Could you check a few things on this model? Use its own coordinates, in mm. Coordinates: 2 decimals unless noted, no trailing zeros. Order: outer loops, then holes, each group sorted by start corner. A loop starts at its lowest first (then second) coordinate and runs counter-clockwise, first axis right, second up. Notation, with made-up numbers: (19.25, 14.5) - (68.25, 14.5) arc R23 cw to (68.25, 26.5) - close; hole circle Ø4 at (-38, -23.5). An arc over 180 degrees is marked (long way). One line per item, written item: value.
from build123d import *

# Parameters (mm, degrees)
EXTRUDE_1_DEPTH     = 2
FILLET_1_R          = 5
FILLET_2_R          = 2
SKETCH_2_R          = 1.55
CUT_EXTRUDE_1_DEPTH = 2


with BuildPart() as part:
    # 草图1 → 凸台-拉伸1 (new body)
    with BuildSketch(Plane.XY):
        Polygon((387.201278127, -62.835808376), (387.201278127, 41.164191624), (257.201278127, 41.164191624), (213.03572495, 25.089244888), (173.136911199, -10.835808376), (213.03572495, -46.760861639), (257.201278127, -62.835808376), align=None)
    extrude(amount=EXTRUDE_1_DEPTH)

    # 圆角1
    fillet_1_edges = [part.edges().sort_by_distance(p)[0] for p in [
        (173.136911199, -10.835808376, 1),
    ]]
    fillet(fillet_1_edges, radius=FILLET_1_R)

    # 圆角2
    fillet_2_edges = [part.edges().sort_by_distance(p)[0] for p in [
        (257.201278127, -62.835808376, 1),
        (213.03572495, -46.760861639, 1),
        (213.03572495, 25.089244888, 1),
        (257.201278127, 41.164191624, 1),
        (387.201278127, 41.164191624, 1),
        (387.201278127, -62.835808376, 1),
    ]]
    fillet(fillet_2_edges, radius=FILLET_2_R)

    # 草图2 → 切除-拉伸1 (cut)
    with BuildSketch(Plane(origin=(0, 0, 0), x_dir=(-1, 0, 0), z_dir=(0, 0, -1))):
        with Locations((-265.201278127, 36.164191624)):
            Circle(SKETCH_2_R)
        with Locations((-251.041024089, 31.834064606)):
            Circle(SKETCH_2_R)
        with Locations((-336.201278127, 26.164191624)):
            Circle(SKETCH_2_R)
        with Locations((-265.201278127, 26.164191624)):
            Circle(SKETCH_2_R)
        with Locations((-265.201278127, -0.835808376)):
            Circle(SKETCH_2_R)
        with Locations((-382.201278127, 36.164191624)):
            Circle(SKETCH_2_R)
        with Locations((-382.201278127, 26.164191624)):
            Circle(SKETCH_2_R)
        with Locations((-196.481423651, 0.334064606)):
            Circle(SKETCH_2_R)
        with Locations((-326.201278127, -10.835808376)):
            Circle(SKETCH_2_R)
        with Locations((-196.201278127, -10.835808376)):
            Circle(SKETCH_2_R)
        with Locations((-196.481423651, -22.005681357)):
            Circle(SKETCH_2_R)
        with Locations((-265.201278127, -20.835808376)):
            Circle(SKETCH_2_R)
        with Locations((-265.201278127, -57.835808376)):
            Circle(SKETCH_2_R)
        with Locations((-265.201278127, -47.835808376)):
            Circle(SKETCH_2_R)
        with Locations((-336.201278127, -47.835808376)):
            Circle(SKETCH_2_R)
        with Locations((-382.201278127, -47.835808376)):
            Circle(SKETCH_2_R)
        with Locations((-382.201278127, -57.835808376)):
            Circle(SKETCH_2_R)
        with Locations((-265.201278127, -10.835808376)):
            Circle(SKETCH_2_R)
        with Locations((-336.201278127, 36.164191624)):
            Circle(SKETCH_2_R)
        with Locations((-336.201278127, -57.835808376)):
            Circle(SKETCH_2_R)
        with Locations((-251.041024089, -53.505681357)):
            Circle(SKETCH_2_R)
        with Locations((-382.201278127, 16.164191624)):
            Circle(SKETCH_2_R)
        with Locations((-382.201278127, -37.835808376)):
            Circle(SKETCH_2_R)
    extrude(amount=-CUT_EXTRUDE_1_DEPTH, mode=Mode.SUBTRACT)


solid = part.part
Item 1: I want a section at B-B on x = 191.5. Please give me the cut outline in (y, z), then the cut area to 3 significant figures.
Conclusion:
outline: (-27.37, 0) - (5.7, 0) - (5.7, 2) - (-27.37, 2) - close
area: 66.1 mm²
Item 2: I want a section at C-C on y = 7. Please give me the cut outline in (x, z).
Conclusion:
outline: (192.95, 0) - (387.2, 0) - (387.2, 2) - (192.95, 2) - close
Item 3: If I drill on probe 1 along Y at (x, z) = (326, 1.35); probe 2 along X at (y, z) = (0.5, 1.85); probe 3 along X at (y, z) = (-22, 1), over which ranges is the centre line in solid material (lowest first)?
Conclusion:
probe 1: -62.84 to -12.37, -9.3 to 41.16
probe 2: 185.73 to 194.94, 198.02 to 264.42, 265.99 to 387.2
probe 3: 185.54 to 194.93, 198.03 to 264.18, 266.22 to 387.2
Item 4: I want a section at A-A on z = 0.85. Give the number of separate pieces and of enclosed holes in the cut face, then the cut area to 3 significant figures.
Conclusion:
separate pieces: 1
enclosed holes: 23
area: 18,700 mm²
